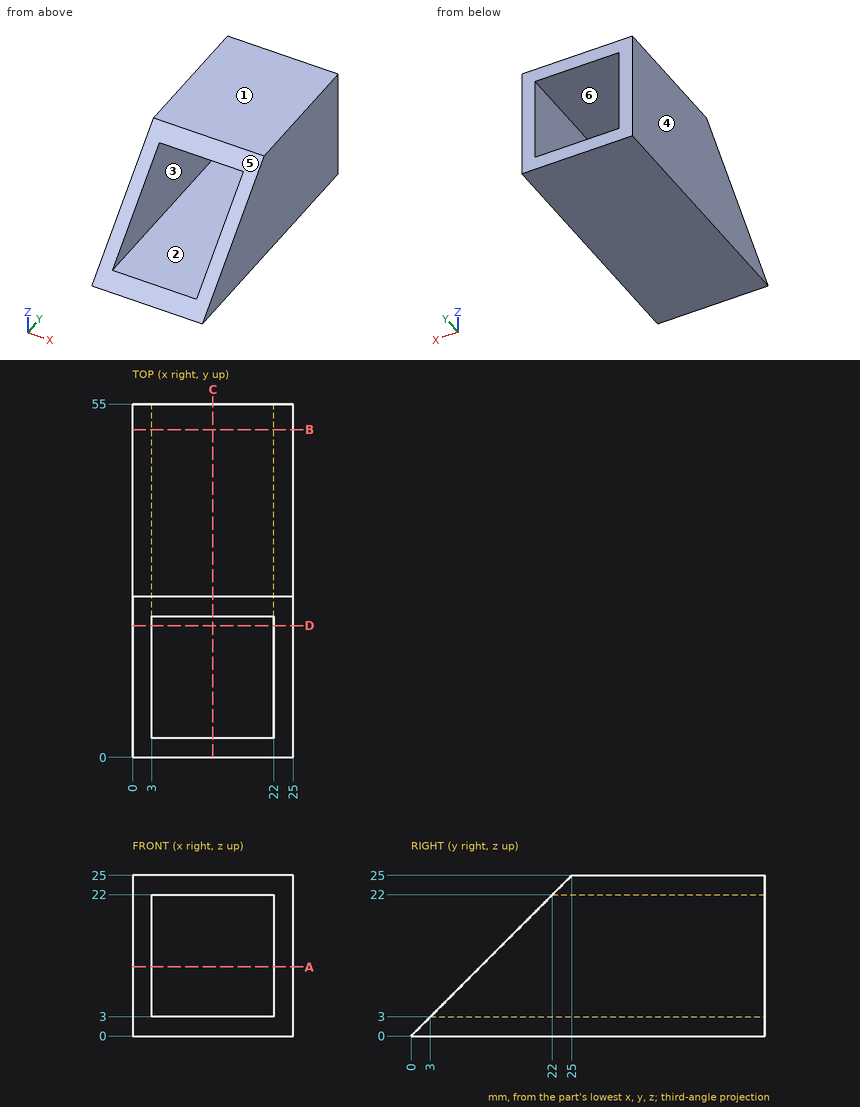
Part print with two shaded views. Sizes in mm from the minimum x, y, z corner. A direction names the side the tool comes from. Round coordinates to 2 decimals unless told otherwise and drop trailing zeros. Order: outer loops, then holes, each group sorted by start corner. A loop starts at its lowest first (then second) coordinate and runs counter-clockwise, first axis right, second up. Notation, with made-up numbers: M 78,78.25 L 128,78.25 A19 cw 128,84.25 Z; hole C -32,-23.5 d9. An arc over 180 degrees is marked long. Put each result on its own line as item: value. Start each with the question number.
1. Drill centre lines: probe 1 along Z at (x, y) = (12, 29); probe 2 along Z at (x, y) = (14.5, 17). Where is each one in solid material? Low to high. Write a range as [from, to].
2. Two-plate mould, pull along X, no slides. Class the marked faces 1, 2, 3 and 4: +X half, -X half, draft (parallel to the pull), parting line (faces both ways), or undercut.
3. Slice it at A-A on z = 10.75. List the corners of the cut face in (x, y).
4. Slice it at C-C on x = 12.5. List the corners of the cut face in (y, z), then the cut area to 3 significant figures.
5. Slice it at B-B on y = 51. List the corners of the cut face in (x, z).
6. Tool access for the marked faces 5 and 6: list every direction of +Z, -Z, +X, -X, +Y, -Y with a clear straight run to the whole face (end or side of a thin tool).
7. Drop a flat-ended pin along its axis: pin 1 (8 mm diameter, centred on x = 13.5, y = 6, fed in from +Z). Give the stop position or say it passes through.
8. Slice it at D-D on y = 20.5. List the corners of the cut face in (x, z).
Findings:
1. probe 1: [0, 3], [22, 25]
1. probe 2: [0, 3]
2. face 1: draft
2. face 2: undercut
2. face 3: undercut
2. face 4: -X half
3. outline: M 0,10.75 L 3,10.75 L 3,55 L 0,55 Z; M 22,10.75 L 25,10.75 L 25,55 L 22,55 Z
4. outline: M 0,0 L 55,0 L 55,3 L 3,3 Z; M 22,22 L 55,22 L 55,25 L 25,25 Z
4. area: 255 mm2
5. outline: M 0,0 L 25,0 L 25,25 L 0,25 Z; hole M 3,3 L 22,3 L 22,22 L 3,22 Z
6. face 5: +Z, +X, -X, -Y
6. face 6: +Y, -Y
7. pin 1: z = 3
8. outline: M 0,0 L 25,0 L 25,20.5 L 22,20.5 L 22,3 L 3,3 L 3,20.5 L 0,20.5 Z
